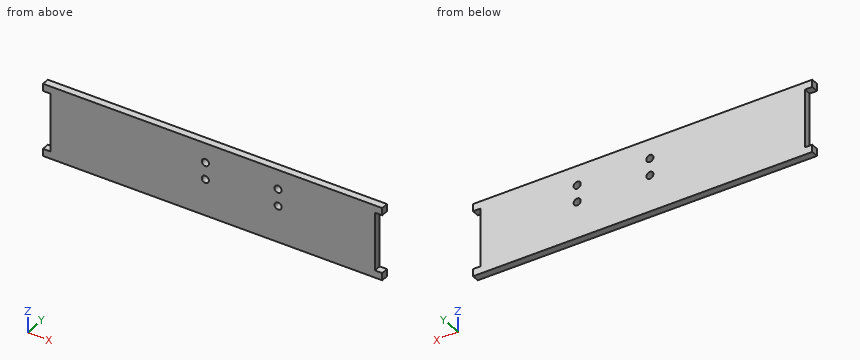
from build123d import *

# Parameters (mm, degrees)
SKETCH1_W           = 140
SKETCH1_H           = 30
BOSS_EXTRUDE1_DEPTH = 3
SKETCH2_W           = 3
SKETCH2_H           = 24
CUT_EXTRUDE1_DEPTH  = 3
SKETCH3_R           = 1.47
CUT_EXTRUDE2_DEPTH  = 3


with BuildPart() as part:
    # Sketch1 → Boss-Extrude1 (new body)
    with BuildSketch(Plane(origin=(0, 0, 0), x_dir=(1, 0, 0), z_dir=(0, 1, 0))):
        Rectangle(SKETCH1_W, SKETCH1_H)
    extrude(amount=BOSS_EXTRUDE1_DEPTH)

    # Sketch2 → Cut-Extrude1 (cut)
    with BuildSketch(Plane(origin=(0, 3, 0), x_dir=(1, 0, 0), z_dir=(0, 1, 0))):
        with Locations((-68.5, 0)):
            Rectangle(SKETCH2_W, SKETCH2_H)
        with Locations((68.5, 0)):
            Rectangle(SKETCH2_W, SKETCH2_H)
    extrude(amount=-CUT_EXTRUDE1_DEPTH, mode=Mode.SUBTRACT)

    # Sketch3 → Cut-Extrude2 (cut)
    with BuildSketch(Plane(origin=(0, 3, 0), x_dir=(1, 0, 0), z_dir=(0, 1, 0))):
        with Locations((-3, 0)):
            Circle(SKETCH3_R)
        with Locations((-3, -7)):
            Circle(SKETCH3_R)
        with Locations((27, 0)):
            Circle(SKETCH3_R)
        with Locations((27, -7)):
            Circle(SKETCH3_R)
    extrude(amount=-CUT_EXTRUDE2_DEPTH, mode=Mode.SUBTRACT)


solid = part.part
Check sheet for the modelled part. Datum: model origin and axes. Units: mm. Give positions to 0.01 mm unless a question says otherwise; leave off trailing zeros. Loops run counter-clockwise (first coordinate to the right, second up) from the corner with the lowest first, then second, coordinate; pieces in that order, holes last. Notation, with made-up numbers: M -1.75,33 L 33.25,33 A24 cw 33.25,49 Z; hole C 86.25,55.5 d2. An arc over 180 degrees is marked long. Return JSON: item names as keys, results as strings. Group by question number.
1. Thickness scan on L1, parallel to Z at x = 27, y = 1.4; L2, parallel to X at y = 1.95, z = 7; L3, parallel to X at y = 0.6, z = -8. Record the ranges inside material, lowest first.
2. Cross-section at C-C on y = 1.45. Record the boundary of the cut face in (x, z).
3. Cross-section at A-A on x = 27. Record the boundary of the cut face in (y, z).
4. Cross-section at B-B on z = 7. Record the boundary of the cut face in (x, y), plus the area to 3 significant figures.
Return value:
{
 "1": {"L1": "-15 to -1.47, 1.47 to 5.53, 8.47 to 15", "L2": "-67 to -4.47, -1.53 to 25.53, 28.47 to 67", "L3": "-67 to 67"},
 "2": {"outline": "M -70,-15 L 70,-15 L 70,-12 L 67,-12 L 67,12 L 70,12 L 70,15 L -70,15 L -70,12 L -67,12 L -67,-12 L -70,-12 Z; hole C -3,0 d2.94; hole C -3,7 d2.94; hole C 27,0 d2.94; hole C 27,7 d2.94"},
 "3": {"outline": "M 0,-15 L 3,-15 L 3,-1.47 L 0,-1.47 Z; M 0,1.47 L 3,1.47 L 3,5.53 L 0,5.53 Z; M 0,8.47 L 3,8.47 L 3,15 L 0,15 Z"},
 "4": {"outline": "M -67,0 L -4.47,0 L -4.47,3 L -67,3 Z; M -1.53,0 L 25.53,0 L 25.53,3 L -1.53,3 Z; M 28.47,0 L 67,0 L 67,3 L 28.47,3 Z", "area": "384 mm^2"}
}
